from build123d import *

# Parameters (mm, degrees)
SKETCH014_R     = 3.75
POCKET006_DEPTH = 9.70192
CHAMFER007_SIZE = 0.4
CHAMFER006_SIZE = 0.1


with BuildPart() as pocket006:
    # Sketch015 → Revolution006 (revolve)
    with BuildSketch(Plane.XZ):
        Polygon((0, 0.29908), (2.75, 1.3), (2.75, 10), (0, 10), align=None)
    revolve(axis=Axis((0, 0, 0), (0, 0, 1)))

    # Sketch014 (on Face3 of Revolution006) → Pocket006 (cut, through all)
    with BuildSketch(Plane(origin=(0, 0, 10), x_dir=(-1, 0, 0), z_dir=(0, 0, 1))):
        Circle(SKETCH014_R)
        Polygon((-0.721688, 1.25), (0.721688, 1.25), (1.443376, 0), (0.721688, -1.25), (-0.721688, -1.25), (-1.443376, 0), align=None, mode=Mode.SUBTRACT)
    extrude(amount=-POCKET006_DEPTH, mode=Mode.SUBTRACT)


with BuildPart() as chamfer006:
    # Sketch016 → Revolution007 (revolve)
    with BuildSketch(Plane.XZ):
        Polygon((1.45, 3), (2.75, 3), (2.75, 0), (1.5, 0), (1.5, -12), (0, -12), (0, 1.549999), align=None)
    revolve(axis=Axis((0, 0, 0), (0, 0, 1)))

    # Cut003: cut Pocket006
    add(pocket006.part, mode=Mode.SUBTRACT)

    # Chamfer007
    chamfer007_edges = [chamfer006.edges().sort_by_distance(p)[0] for p in [
        (-1.5, 0, -12),
    ]]
    chamfer(chamfer007_edges, length=CHAMFER007_SIZE)

    # Chamfer006
    chamfer006_edges = [chamfer006.edges().sort_by_distance(p)[0] for p in [
        (-2.75, 0, 0),
        (-2.75, 0, 3),
    ]]
    chamfer(chamfer006_edges, length=CHAMFER006_SIZE)


solid = chamfer006.part
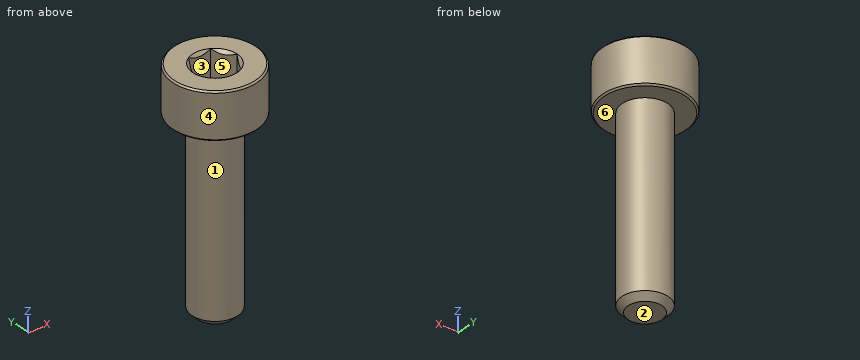
Geometry check sheet. Reference: the model listing, model coordinates, mm. Face numbers are marked on the shaded views. A direction names the side the tool comes from. Coordinates: 2 decimals unless noted, no trailing zeros. Loops run counter-clockwise (first coordinate to the right, second up) from the corner with the lowest first, then second, coordinate; pieces in that order, holes last. Notation, with made-up numbers: (14.25, -8) - (29.25, -8) arc R26 ccw to (29.25, 19) - close; hole circle Ø4 at (-6, 12). An arc over 180 degrees is marked (long way). Use one line per item in the form item = value. Start each with the question number.
Item 1: Gauge pin test, flat ends, axial feed: pin 1 (0.7 mm diameter, centred on x = -0.5, z = 2.5, fed in from +Y); pin 2 (1.5 mm diameter, centred on y = -2, z = -4, fed in from -X). Record the tip position at first contact, or that the pin passes through.
Item 2: Mould release check, pull along Y, two halves, no side actions. Record for the marked faces 1, 2 and 3: +Y half, -Y half, draft (parallel to the pull), parting line (faces both ways), or undercut.
Item 3: Tool access check on the marked faces 4, 5 and 6. Record the directions out of +Z, -Z, +X, -X, +Y, -Y that give a thin tool (end or side, any length) a straight path to the whole face; none if there is none.
Item 4: Section check A-A, the plane z = 1.75. Enter the section's corners in (x, y).
Item 5: Section check B-B, the plane z = -9.5. Enter the section's corners in (x, y).
Item 6: Thickness scan on probe 1 along Y at (x, z) = (-0.05, -2.75); probe 2 along Z at (x, y) = (-0.7, -2.25); probe 3 along Y at (x, z) = (0.65, -6). Record the ranges inside material, lowest first.
Computed:
q1.pin_1 = 2.75
q1.pin_2 = -0.83
q2.face_1 = parting line
q2.face_2 = draft
q2.face_3 = undercut
q3.face_4 = +Z, -Z
q3.face_5 = +Z
q3.face_6 = -Z
q4.outline = circle Ø5.5 at (0, 0); hole (-1.44, 0) - (-0.72, -1.25) - (0.72, -1.25) - (1.44, 0) - (0.72, 1.25) - (-0.72, 1.25) - close
q5.outline = circle Ø3 at (0, 0)
q6.probe_1 = -1.5 to 1.5
q6.probe_2 = 0 to 3
q6.probe_3 = -1.35 to 1.35
